Build history of the part. All positions in model axes, mm. Face numbers are marked on the shaded views. A direction names the side the tool comes from. Give positions to 0.01 mm unless a question says otherwise; leave off trailing zeros. Order: outer loops, then holes, each group sorted by start corner. A loop starts at its lowest first (then second) coordinate and runs counter-clockwise, first axis right, second up. Notation, with made-up numbers: M -34.5,36.25 L 23.5,36.25 A31 cw 23.5,66.25 Z; hole C 82.25,87.25 d4. An arc over 180 degrees is marked long. One line per item, written item: value.
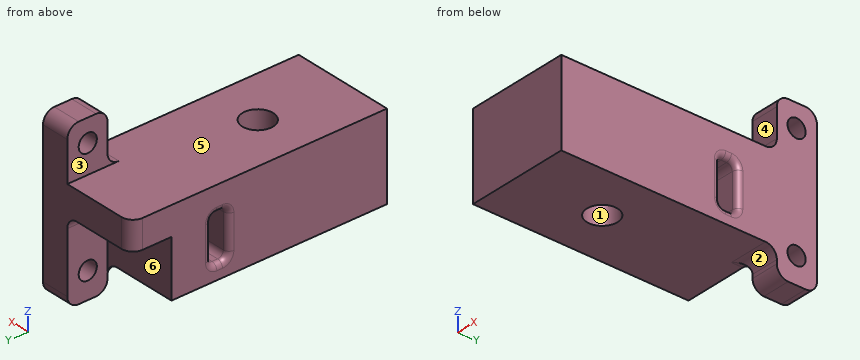
from build123d import *

# Parameters (mm, degrees)
SKETCH1_W           = 23.056445047489827
SKETCH1_H           = 95.25
SKETCH1_R           = 1.2700000000000005
SKETCH1_R_2         = 1.269999999999998
BOSS_EXTRUDE1_DEPTH = 6.35
SKETCH2_W           = 23.056445047489827
SKETCH2_H           = 48.26
BOSS_EXTRUDE2_DEPTH = 12.7
CUT_EXTRUDE2_DEPTH  = 55.41534970233967
SKETCH6_R           = 3.4289999999999994
CUT_EXTRUDE3_DEPTH  = 53.57321599024526
FILLET2_R           = 1.27
BOSS_EXTRUDE3_DEPTH = 6.35
SKETCH9_R           = 1.9049999999999996
SKETCH9_R_2         = 1.905
CUT_EXTRUDE4_DEPTH  = 53.43149307056342
FILLET4_R           = 2.54
BOSS_EXTRUDE7_DEPTH = 6.35
FILLET5_R           = 2.54
FILLET6_R           = 2.54
SKETCH13_R          = 2.0319999999999987
SKETCH13_R_2        = 2.032000000000001
CUT_EXTRUDE5_DEPTH  = 6.35
FILLET7_R           = 2.54
SKETCH14_W          = 8.8077942060624
SKETCH14_H          = 39.07493764297598
CUT_EXTRUDE6_DEPTH  = 45.21200000000002
SKETCH15_W          = 6.35
SKETCH15_H          = 6.35
CUT_EXTRUDE7_DEPTH  = 7.112000000000007
FILLET8_R           = 2.54


with BuildPart() as part:
    # Sketch1 → Boss-Extrude1 (new body)
    # profile 1 of 4: a face of its own
    with BuildSketch(Plane.XY):
        Rectangle(SKETCH1_W, SKETCH1_H)
        Polygon((7.9121000000000015, 16.687800000000006), (7.9121000000000015, 44.449999999999996), (-7.912099999999998, 44.45), (-7.912099999999998, 16.687800000000006), align=None, mode=Mode.SUBTRACT)
    # profile 2 of 4: a face of its own
    with BuildSketch(Plane.XY):
        Polygon((-7.912099999999998, 16.687800000000006), (7.9121000000000015, 16.687800000000006), (7.9121000000000015, 44.449999999999996), (-7.912099999999998, 44.45), align=None)
        with Locations((5.372100000000001, 19.227800000000006)):
            Circle(SKETCH1_R, mode=Mode.SUBTRACT)
        with Locations((-5.372099999999998, 41.910000000000004)):
            Circle(SKETCH1_R_2, mode=Mode.SUBTRACT)
    # profile 3 of 4: a face of its own
    with BuildSketch(Plane.XY):
        with Locations((-5.372099999999998, 41.910000000000004)):
            Circle(SKETCH1_R_2)
    # profile 4 of 4: a face of its own
    with BuildSketch(Plane.XY):
        with Locations((5.372100000000001, 19.227800000000006)):
            Circle(SKETCH1_R)
    extrude(amount=BOSS_EXTRUDE1_DEPTH)

    # Sketch2 → Boss-Extrude2 (add)
    with BuildSketch(Plane(origin=(0, 0, 0), x_dir=(-1, 0, 0), z_dir=(0, 0, -1))):
        with Locations((0, -23.495)):
            Rectangle(SKETCH2_W, SKETCH2_H)
    extrude(amount=BOSS_EXTRUDE2_DEPTH)

    # Sketch5 → Cut-Extrude2 (cut, through all)
    with BuildSketch(Plane(origin=(11.528222523744914, 0, 0), x_dir=(0, 0, -1), z_dir=(1, 0, 0))):
        Polygon((-0.6350000000000019, -12.065000000000001), (9.524999999999997, -12.065000000000001), (9.524999999999999, -8.255000000000003), (-0.6350000000000019, -8.255000000000003), align=None)
    extrude(amount=-CUT_EXTRUDE2_DEPTH, mode=Mode.SUBTRACT)

    # Sketch6 → Cut-Extrude3 (cut, through all)
    with BuildSketch(Plane(origin=(0, 0, -12.7), x_dir=(-1, 0, 0), z_dir=(0, 0, -1))):
        with Locations((0, -28.575)):
            Circle(SKETCH6_R)
    extrude(amount=-CUT_EXTRUDE3_DEPTH, mode=Mode.SUBTRACT)

    # Fillet2
    fillet2_edges = [part.edges().sort_by_distance(p)[0] for p in [
        (-11.528222523744914, -10.160000000000004, -9.524999999999999),
        (0, -8.255000000000003, -9.524999999999999),
        (-11.528222523744914, -12.065, -4.444999999999998),
        (0, -12.065000000000001, -9.524999999999997),
        (-11.528222523744914, -10.16, 0.6350000000000019),
        (0, -12.065000000000001, 0.6350000000000019),
        (-11.528222523744914, -8.255000000000003, -4.4449999999999985),
        (0, -8.255000000000003, 0.6350000000000019),
        (11.528222523744914, -10.160000000000002, -9.524999999999999),
        (11.528222523744914, -8.255000000000003, -4.4449999999999985),
        (11.528222523744914, -10.160000000000002, 0.6350000000000019),
        (11.528222523744914, -12.065000000000001, -4.444999999999998),
    ]]
    fillet(fillet2_edges, radius=FILLET2_R)

    # Sketch8 → Boss-Extrude3 (add)
    with BuildSketch(Plane.ZY.offset(11.528222523744914)):
        Polygon((6.35, 47.625), (-1.21e-15, 47.625), (0, 6.98625472546675), (6.350000000000005, 6.986254725466751), align=None)
    extrude(amount=BOSS_EXTRUDE3_DEPTH)

    # Sketch9 → Cut-Extrude4 (cut, through all)
    with BuildSketch(Plane.XY):
        with Locations((-4.594022523744915, 12.877800000000006)):
            Circle(SKETCH9_R)
        with Locations((-15.338222523744914, 35.56)):
            Circle(SKETCH9_R_2)
    extrude(amount=CUT_EXTRUDE4_DEPTH, mode=Mode.SUBTRACT)

    # Fillet4
    fillet4_edges = [part.edges().sort_by_distance(p)[0] for p in [
        (11.528222523744914, 47.625, 3.175),
        (-17.878222523744913, 47.625, 3.1749999999999994),
    ]]
    fillet(fillet4_edges, radius=FILLET4_R)

    # Sketch12 → Boss-Extrude7 (add)
    with BuildSketch(Plane(origin=(11.528222523744914, 0, 0), x_dir=(0, 0, -1), z_dir=(1, 0, 0))):
        Polygon((-6.35, 0.6349999999999898), (18.613653389650153, 0.6349999999999898), (18.613653389650153, 9.627193152709879), (-17.78195834691587, 9.627193152709879), (-17.78195834691587, 0.6349999999999898), align=None)
    extrude(amount=-BOSS_EXTRUDE7_DEPTH)

    # Fillet5
    fillet5_edges = [part.edges().sort_by_distance(p)[0] for p in [
        (8.353222523744913, 0.6349999999999967, -12.7),
        (5.178222523744914, 5.131096576354938, 0),
        (8.353222523744915, 0.6349999999999898, 6.35),
    ]]
    fillet(fillet5_edges, radius=FILLET5_R)

    # Fillet6
    fillet6_edges = [part.edges().sort_by_distance(p)[0] for p in [
        (5.178222523744914, -0.6350000000000069, -12.7),
    ]]
    fillet(fillet6_edges, radius=FILLET6_R)

    # Sketch13 → Cut-Extrude5 (cut)
    with BuildSketch(Plane(origin=(11.528222523744914, 0, 0), x_dir=(0, 0, -1), z_dir=(1, 0, 0))):
        with Locations((-12.70195834691587, 5.050717249087455)):
            Circle(SKETCH13_R)
        with Locations((12.698041653084129, 5.050717249087455)):
            Circle(SKETCH13_R_2)
    extrude(amount=-CUT_EXTRUDE5_DEPTH, mode=Mode.SUBTRACT)

    # Fillet7
    fillet7_edges = [part.edges().sort_by_distance(p)[0] for p in [
        (8.353222523744915, 0.6349999999999898, -18.613653389650153),
        (8.353222523744915, 0.6349999999999898, 17.78195834691587),
        (8.353222523744915, 9.627193152709879, 17.78195834691587),
        (8.353222523744915, 9.627193152709879, -18.613653389650153),
    ]]
    fillet(fillet7_edges, radius=FILLET7_R)

    # Sketch14 → Cut-Extrude6 (cut)
    with BuildSketch(Plane(origin=(11.528222523744914, 0, 0), x_dir=(0, 0, -1), z_dir=(1, 0, 0))):
        with Locations((-1.9461028969687981, 29.16466197419787)):
            Rectangle(SKETCH14_W, SKETCH14_H)
    extrude(amount=-CUT_EXTRUDE6_DEPTH, mode=Mode.SUBTRACT)

    # Sketch15 → Cut-Extrude7 (cut)
    with BuildSketch(Plane.XZ.offset(-6.98625472546675)):
        with Locations((-14.703222523744913, 3.1750000000000007)):
            Rectangle(SKETCH15_W, SKETCH15_H)
    extrude(amount=-CUT_EXTRUDE7_DEPTH, mode=Mode.SUBTRACT)

    # Fillet8
    fillet8_edges = [part.edges().sort_by_distance(p)[0] for p in [
        (-11.528222523744914, 9.627193152709879, 3.1750000000000007),
    ]]
    fillet(fillet8_edges, radius=FILLET8_R)


solid = part.part
1) Tool access for the marked faces 4, 5 and 6: list every direction of +Z, -Z, +X, -X, +Y, -Y with a clear straight run to the whole face (end or side of a thin tool).
Check values:
face 4: +Z, +X, -X, -Y
face 5: +Z, -X, -Y
face 6: -Z, -X, +Y
2) Drill centre lines: probe 1 along Y at (x, z) = (0, -1.25) (3 decimals); probe 2 along Y at (x, z) = (0, 0.25) (3 decimals); probe 3 along Y at (x, z) = (9.5, -12.5) (3 decimals). Where is each one in solid material? Low to high. Write a range as from..to.
Check values:
probe 1: -47.625..-32.004, -25.146..-12.065, -8.255..0.635
probe 2: -47.625..-32.004, -25.146..-11.706, -8.614..9.627
probe 3: -47.625..3.028, 7.073..9.627
3) Saw through at C-C, the plane y = -44. Write the cut outline in (x, z), then the cut area to 3 significant figures.
Check values:
outline: M -11.53,-12.7 L 11.53,-12.7 L 11.53,6.35 L -11.53,6.35 Z
area: 439 mm^2
4) Saw through at A-A, the plane x = 0. Write the cut outline in (y, z) (3 decimals), then the cut area to 3 significant figures.
Check values:
outline: M -47.625,-12.7 L -32.004,-12.7 L -32.004,6.35 L -47.625,6.35 Z; M -25.146,-12.7 L 0.635,-12.7 L 0.635,0 L 9.627,0 L 9.627,6.35 L -25.146,6.35 Z; hole M -12.065,-8.255 A1.27 ccw -10.795,-9.525 L -9.525,-9.525 A1.27 ccw -8.255,-8.255 L -8.255,-0.635 A1.27 ccw -9.525,0.635 L -10.795,0.635 A1.27 ccw -12.065,-0.635 Z
area: 808 mm^2
5) Saw through at B-B, the plane z = -14. Write the cut outline in (x, y) (3 decimals), then the cut area to 3 significant figures.
Check values:
outline: M 4.855,0.312 L 11.528,0.312 L 11.528,3.491 L 5.178,3.491 L 5.178,0.635 L 4.855,0.635 Z; M 5.178,6.611 L 11.528,6.611 L 11.528,9.627 L 5.178,9.627 Z
area: 39.4 mm^2
6) Saw through at D-D, the plane z = 7.5. Write the cut outline in (x, y).
Check values:
outline: M 5.18,0.22 L 11.53,0.22 L 11.53,9.63 L 5.18,9.63 Z
7) Pin check, flat tips, straight feed: pin 1 (0.9 mm diameter, centred on x = 7, z = -15.5, fed in from -Y); pin 2 (5.5 mm diameter, centred on y = 2.5, z = 14.5, fed in from -X); pin 3 (4 mm diameter, centred on x = 1, z = -2.5, fed in from +Y) (3 decimals). Stop position of each tip, or through.
Check values:
pin 1: y = 0.63
pin 2: x = 5.18
pin 3: y = 0.635
8) Mould opens along X. For the marked faces 1, 2 and 3 say: released by +X, released by -X, zero draft, split by the parting line, or undercut.
Check values:
face 1: undercut
face 2: zero draft
face 3: released by -X
